The listing builds one solid part. Answer for the finished solid, in the listing's coordinates (mm). Face numbers are marked on the shaded views. A direction names the side the tool comes from. Coordinates: 2 decimals unless noted, no trailing zeros. Order: outer loops, then holes, each group sorted by start corner. A loop starts at its lowest first (then second) coordinate and runs counter-clockwise, first axis right, second up. Notation, with made-up numbers: (-12, 34.5) -> (45, 34.5) arc R35 cw to (45, 66.5) -> close; hole circle Ø7 at (-4, -28). An arc over 180 degrees is marked (long way). Write item = value, one per line. Start each with the question number.
```python
from build123d import *

# Parameters (mm, degrees)
SKETCH_1_W          = 58
SKETCH_1_H          = 58
EXTRUDE_1_DEPTH     = 4
SKETCH_6_R          = 19.5
SKETCH_6_R_2        = 2.6
CUT_EXTRUDE_1_DEPTH = 42.206795556
SKETCH_3_W          = 70
SKETCH_3_H          = 40
EXTRUDE_2_DEPTH     = 8
EXTRUDE_3_DEPTH     = 6
SKETCH_8_R          = 2.6
CUT_EXTRUDE_2_DEPTH = 72.224995612
SKETCH_9_R          = 5
CUT_EXTRUDE_3_DEPTH = 3
CHAMFER_2_SIZE      = 3
CHAMFER_1_SIZE      = 3
SKETCH_11_R         = 5
CUT_EXTRUDE_4_DEPTH = 56.479726027


with BuildPart() as part:
    # Эскиз1 → Бобышка-Вытянуть1 (new body)
    with BuildSketch(Plane.XY):
        Rectangle(SKETCH_1_W, SKETCH_1_H)
    extrude(amount=EXTRUDE_1_DEPTH)

    # Эскиз6 → Вырез-Вытянуть1 (cut, through all)
    with BuildSketch(Plane.XY.offset(4)):
        Circle(SKETCH_6_R)
        with Locations((-23.57, 23.57)):
            Circle(SKETCH_6_R_2)
        with Locations((23.57, 23.57)):
            Circle(SKETCH_6_R_2)
        with Locations((-23.57, -23.57)):
            Circle(SKETCH_6_R_2)
        with Locations((23.57, -23.57)):
            Circle(SKETCH_6_R_2)
    extrude(amount=-CUT_EXTRUDE_1_DEPTH, mode=Mode.SUBTRACT)

    # Эскиз3 → Бобышка-Вытянуть2 (add)
    with BuildSketch(Plane(origin=(0, 29, 0), x_dir=(1, 0, 0), z_dir=(0, 1, 0))):
        with Locations((0, -2)):
            Rectangle(SKETCH_3_W, SKETCH_3_H)
    extrude(amount=EXTRUDE_2_DEPTH)

    # Эскиз5 → Бобышка-Вытянуть3 (add)
    with BuildSketch(Plane(origin=(29, 0, 0), x_dir=(0, 0, -1), z_dir=(1, 0, 0))):
        Polygon((-4, -29), (0, -29), (18, 29), (-22, 29), align=None)
    extrude_3 = extrude(amount=EXTRUDE_3_DEPTH)

    # Зеркальное отражение3: Бобышка-Вытянуть3 across plane
    add(extrude_3.mirror(Plane(origin=(0, 0, 0), x_dir=(0, 0, 1), z_dir=(1, 0, 0))))

    # Эскиз8 → Вырез-Вытянуть2 (cut, through all)
    with BuildSketch(Plane(origin=(0, 29, 0), x_dir=(1, 0, 0), z_dir=(0, 1, 0))):
        with Locations((18.5, 8)):
            Circle(SKETCH_8_R)
        with Locations(Location((-18.5, 8, 0), (0, 0, 180))):
            Circle(SKETCH_8_R)
        with Locations(Location((18.5, -12, 0), (0, 0, 180))):
            Circle(SKETCH_8_R)
        with Locations((-18.5, -12)):
            Circle(SKETCH_8_R)
    extrude(amount=CUT_EXTRUDE_2_DEPTH, mode=Mode.SUBTRACT)

    # Эскиз9 → Вырез-Вытянуть3 (cut)
    with BuildSketch(Plane.XZ.offset(-29)):
        with Locations((-18.5, -8)):
            Circle(SKETCH_9_R)
        with Locations((18.5, -8)):
            Circle(SKETCH_9_R)
    extrude(amount=-CUT_EXTRUDE_3_DEPTH, mode=Mode.SUBTRACT)

    # Фаска2
    # the kernel refuses this chamfer: 3 mm, written as the material it adds along each edge
    with BuildSketch(Plane(origin=(29, -29, 4), x_dir=(0.027495876610586775, 0, 0.9996219169112968), z_dir=(0, 1, 0))) as chamfer_2_piece_1_section:
        Polygon((CHAMFER_2_SIZE * 0.999621916911, -CHAMFER_2_SIZE * 0.0274958766106), (-CHAMFER_2_SIZE * 0.0274958766106, -CHAMFER_2_SIZE * 0.999621916911), (0, 0), align=None)
    chamfer_2_piece_1 = extrude(amount=65.715048964, mode=Mode.PRIVATE)
    chamfer_2_piece_1 = split(chamfer_2_piece_1, bisect_by=Plane(origin=(27.993637715, -0.868614474, 12.730429991), z_dir=(0, 0.2963992148724529, -0.9550641368112371)), keep=Keep.TOP, mode=Mode.PRIVATE)
    chamfer_2_piece_1 = chamfer_2_piece_1 - Plane(origin=(23.57, -23.57, 4.956337432), x_dir=(1, 0, 0), z_dir=(0, 0, 1)) * Cylinder(2.6, 144, mode=Mode.PRIVATE)
    chamfer_2_piece_1 = chamfer_2_piece_1 - Plane(origin=(23.57, 23.57, 4.956337432), x_dir=(1, 0, 0), z_dir=(0, 0, 1)) * Cylinder(2.6, 144, mode=Mode.PRIVATE)
    add(chamfer_2_piece_1)
    with BuildSketch(Plane(origin=(-29, 36.715048964, 4), x_dir=(0.9996219169112968, 0, -0.027495876610586334), z_dir=(0, -1, 0))) as chamfer_2_piece_2_section:
        Polygon((CHAMFER_2_SIZE * 0.999621916911, CHAMFER_2_SIZE * 0.0274958766106), (-CHAMFER_2_SIZE * 0.0274958766106, CHAMFER_2_SIZE * 0.999621916911), (0, 0), align=None)
    chamfer_2_piece_2 = extrude(amount=65.715048964, mode=Mode.PRIVATE)
    chamfer_2_piece_2 = split(chamfer_2_piece_2, bisect_by=Plane(origin=(-28.01061912, 27.703260845, 21.597563711), z_dir=(0, 0.2963992148724529, -0.9550641368112371)), keep=Keep.TOP, mode=Mode.PRIVATE)
    chamfer_2_piece_2 = chamfer_2_piece_2 - Plane(origin=(-23.57, -23.57, 4.98938088), x_dir=(1, 0, 0), z_dir=(0, 0, 1)) * Cylinder(2.6, 144, mode=Mode.PRIVATE)
    chamfer_2_piece_2 = chamfer_2_piece_2 - Plane(origin=(-23.57, 23.57, 4.98938088), x_dir=(1, 0, 0), z_dir=(0, 0, 1)) * Cylinder(2.6, 144, mode=Mode.PRIVATE)
    add(chamfer_2_piece_2)

    # Фаска1
    chamfer_1_edges = [part.edges().sort_by_distance(p)[0] for p in [
        (-29, 29, 14.5),
        (29, 29, 14.5),
        (29, 29, -9),
        (-29, 29, -9),
    ]]
    chamfer(chamfer_1_edges, length=CHAMFER_1_SIZE)

    # Эскиз11 → Вырез-Вытянуть4 (cut, through all)
    with BuildSketch(Plane.XY.offset(4)):
        with Locations((-23.57, 23.57)):
            Circle(SKETCH_11_R)
        with Locations((23.57, 23.57)):
            Circle(SKETCH_11_R)
        with Locations((23.57, -23.57)):
            Circle(SKETCH_11_R)
        with Locations((-23.57, -23.57)):
            Circle(SKETCH_11_R)
    extrude(amount=CUT_EXTRUDE_4_DEPTH, mode=Mode.SUBTRACT)


solid = part.part
```
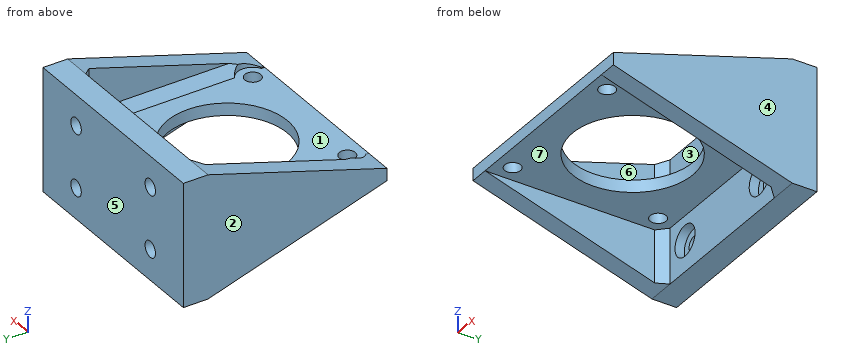
Item 1: Which of the six approach directions +Z, -Z, +X, -X, +Y, -Y give full straight-line access (tool end or side, diameter ignored) to the marked faces 5, 6 and 7?
Item 2: For a pull along X with two mould halves and no side action, classify the marked faces 1, 2, 3 and 4 as pulls with the +X half, pulls with the -X half, needs draft (parallel to the pull), parting line crosses it, or undercut.
Item 3: Each of these flat-tipped pins is pushed along its axis until it touches: pin 1 (4.5 mm diameter, centred on x = -18.5, z = 12, fed in from -Y); pin 2 (13.5 mm diameter, centred on y = -9.5, z = -9, fed in from +X); pin 3 (8 mm diameter, centred on x = 13, y = -18, fed in from +Z); pin 4 (3 mm diameter, centred on x = 20.5, z = -9, fed in from -Y). Where does it stop, or does it pass through?
Item 4: Section D-D, the plane y = -3 is taken. Give the vertices of the cut face in (x, z), then the cut area to 3 significant figures.
Item 5: Section B-B, the plane x = -8 is taken. Give the vertices of the cut face in (y, z).
Item 6: Section C-C, the plane x = 22.5 is taken. Give the vertices of the cut face in (y, z), then the cut area to 3 significant figures.
Item 7: Consider probe 1 along Y at (x, z) = (-23.57, 2.75); probe 2 along Z at (x, y) = (-18.5, 34.5); probe 3 along X at (y, z) = (-1.5, 12). Determine where each line is inside the solid, lowest interval first.
Item 8: Section A-A, the plane z = 13 is taken. Give the vertices of the cut face in (x, y), then the cut area to 3 significant figures.
A:
q1.face_5 = +Z, -Z, +X, -X, +Y
q1.face_6 = +Z, -Y
q1.face_7 = -Z, -Y
q2.face_1 = undercut
q2.face_2 = pulls with the -X half
q2.face_3 = undercut
q2.face_4 = pulls with the +X half
q3.pin_1 = through
q3.pin_2 = 35
q3.pin_3 = 4
q3.pin_4 = 32
q4.outline = (-35, -8.07) -> (-29, -8.07) -> (-29, 0) -> (-19.27, 0) -> (-19.27, 4) -> (-26, 4) -> (-29, 7) -> (-29, 12.07) -> (-35, 12.07) -> close; (19.27, 0) -> (29, 0) -> (29, -8.07) -> (35, -8.07) -> (35, 12.07) -> (29, 12.07) -> (29, 7) -> (26, 4) -> (19.27, 4) -> close
q4.area = 329 mm^2
q5.outline = (-29, 0) -> (-17.78, 0) -> (-17.78, 4) -> (-29, 4) -> close; (17.78, 0) -> (29, 0) -> (29, -18) -> (37, -18) -> (37, 22) -> (29, 22) -> (29, 4) -> (17.78, 4) -> close
q6.outline = (-29, 0) -> (-25.94, 0) -> (-25.94, 4) -> (-29, 4) -> close; (-21.2, 0) -> (21.2, 0) -> (21.2, 4) -> (-21.2, 4) -> close; (25.94, 0) -> (29, 0) -> (29, -5) -> (32, -5) -> (32, -11) -> (29, -11) -> (29, -18) -> (37, -18) -> (37, 22) -> (29, 22) -> (29, 4) -> (25.94, 4) -> close
q6.area = 496 mm^2
q7.probe_1 = -29 to -26.17, -20.97 to 20.97, 26.17 to 37
q7.probe_2 = -18 to -10.6, -5.4 to 9.4, 14.6 to 22
q7.probe_3 = -35 to -29, 29 to 35
q8.outline = (-35, 0) -> (-29, 0) -> (-29, 26) -> (-26, 29) -> (-20.9, 29) -> (-20.9, 37) -> (-35, 37) -> close; (-16.1, 29) -> (16.1, 29) -> (16.1, 37) -> (-16.1, 37) -> close; (20.9, 29) -> (26, 29) -> (29, 26) -> (29, 0) -> (35, 0) -> (35, 37) -> (20.9, 37) -> close
q8.area = 840 mm^2
